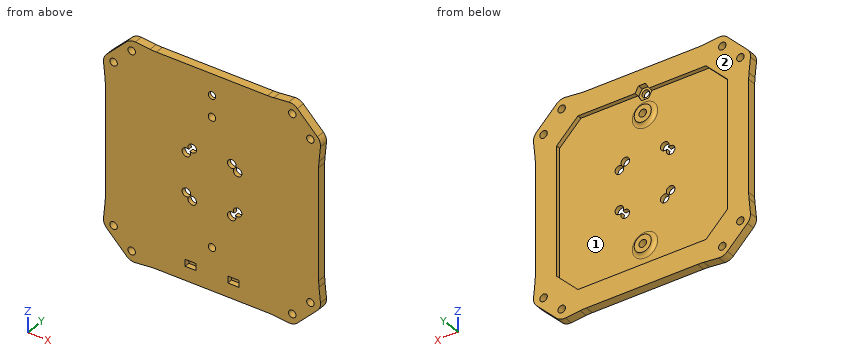
from build123d import *

# Parameters (mm, degrees)
SKETCH1_R                  = 1.75
BOSS_EXTRUDE1_DEPTH        = 4
CUT_EXTRUDE1_DEPTH         = 2
SKETCH4_R                  = 1.75
CUT_EXTRUDE3_DEPTH         = 73.238369544
BOSS_EXTRUDE2_START        = 1.5
SKETCH5_R                  = 4
SKETCH5_R_2                = 1.75
BOSS_EXTRUDE2_DEPTH        = 1.5
REDONDEO1_R                = 2
REDONDEO2_R                = 30
REDONDEO3_R                = 5
CORTAR_EXTRUIR2_DEPTH      = 2.5
CROQUIS1_R                 = 1.75
CORTAR_EXTRUIR1_DEPTH      = 5
CORTAR_EXTRUIR3_DEPTH      = 73.029377138
CORTAR_EXTRUIR3_DEPTH_BACK = 73.029377138
CROQUIS5_R                 = 2
CROQUIS6_W                 = 5.2
CROQUIS6_H                 = 3.2
CORTAR_EXTRUIR4_DEPTH      = 2.5


with BuildPart() as part:
    # Sketch1 → Boss-Extrude1 (new body)
    with BuildSketch(Plane(origin=(0, 0, 0), x_dir=(1, 0, 0), z_dir=(0, 1, 0))):
        Polygon((-27.516424079, 50), (27.516424079, 50), (38.33273811, 51.060660172), (51.060660172, 38.33273811), (50, 27.516424079), (50, -27.516424079), (51.060660172, -38.33273811), (38.33273811, -51.060660172), (27.516424079, -50), (-27.516424079, -50), (-38.33273811, -51.060660172), (-51.060660172, -38.33273811), (-50, -27.516424079), (-50, 27.516424079), (-51.060660172, 38.33273811), (-38.33273811, 51.060660172), align=None)
        with Locations(Location((37.625631329, 46.110912703, 0), (0, 0, 270))):
            Circle(SKETCH1_R, mode=Mode.SUBTRACT)
        with Locations(Location((46.110912703, 37.625631329, 0), (0, 0, 270))):
            Circle(SKETCH1_R, mode=Mode.SUBTRACT)
        with Locations(Location((37.625631329, -46.110912703, 0), (0, 0, 270))):
            Circle(SKETCH1_R, mode=Mode.SUBTRACT)
        with Locations(Location((46.110912703, -37.625631329, 0), (0, 0, 270))):
            Circle(SKETCH1_R, mode=Mode.SUBTRACT)
        with Locations(Location((-46.110912703, -37.625631329, 0), (0, 0, 270))):
            Circle(SKETCH1_R, mode=Mode.SUBTRACT)
        with Locations(Location((-37.625631329, -46.110912703, 0), (0, 0, 270))):
            Circle(SKETCH1_R, mode=Mode.SUBTRACT)
        with Locations(Location((-37.625631329, 46.110912703, 0), (0, 0, 270))):
            Circle(SKETCH1_R, mode=Mode.SUBTRACT)
        with Locations(Location((-46.110912703, 37.625631329, 0), (0, 0, 270))):
            Circle(SKETCH1_R, mode=Mode.SUBTRACT)
    extrude(amount=BOSS_EXTRUDE1_DEPTH)

    # Sketch2 → Cut-Extrude1 (cut)
    with BuildSketch(Plane(origin=(0, 4, 0), x_dir=(1, 0, 0), z_dir=(0, 1, 0))):
        Polygon((-40, -30), (-40, 30), (-30, 40), (30, 40), (40, 30), (40, -30), (30, -40), (-30, -40), align=None)
    extrude(amount=-CUT_EXTRUDE1_DEPTH, mode=Mode.SUBTRACT)

    # Sketch4 → Cut-Extrude3 (cut, through all)
    with BuildSketch(Plane(origin=(0, 2, 0), x_dir=(1, 0, 0), z_dir=(0, 1, 0))):
        with Locations(Location((0, 30, 0), (0, 0, 270))):
            Circle(SKETCH4_R)
    cut_extrude3 = extrude(amount=-CUT_EXTRUDE3_DEPTH, mode=Mode.SUBTRACT)

    # Sketch5 → Boss-Extrude2 (add)
    with BuildSketch(Plane(origin=(0, 2, 0), x_dir=(1, 0, 0), z_dir=(0, 1, 0)).offset(BOSS_EXTRUDE2_START)):
        with Locations(Location((0, 30, 0), (0, 0, 90))):
            Circle(SKETCH5_R)
        with Locations(Location((0, 30, 0), (0, 0, 270))):
            Circle(SKETCH5_R_2, mode=Mode.SUBTRACT)
    boss_extrude2 = extrude(amount=-BOSS_EXTRUDE2_DEPTH)

    # Simetría1: Cut-Extrude3, Boss-Extrude2 across plane
    add(cut_extrude3.mirror(Plane.XY), mode=Mode.SUBTRACT)
    add(boss_extrude2.mirror(Plane.XY))

    # Redondeo1
    # the kernel refuses this fillet: 2 mm, written as the material it adds along each edge
    with BuildSketch(Plane(origin=(0, 2, -30), x_dir=(0, 0, -1), z_dir=(1, 0, 0))) as redondeo1_piece_1:
        with BuildLine():
            CenterArc((5.936491673, 2), REDONDEO1_R, 194.477512186, 75.522487814)
            Line((4, 1.5), (3.961270167, 1.49))
            ThreePointArc((3.961270167, 1.49), (3.96, 0.75), (3.96, 0))
            Line((3.96, 0), (4, -0.04))
            Line((4, -0.04), (5.936491673, -0.04))
            Line((5.936491673, -0.04), (5.936491673, 0))
        make_face()
    revolve(axis=Axis((0, 2, -30), (0, 1, 0)))
    with BuildSketch(Plane(origin=(0, 2, 30), x_dir=(0, 0, 1), z_dir=(1, 0, 0))) as redondeo1_piece_2:
        with BuildLine():
            CenterArc((5.936491673, -2), REDONDEO1_R, 90, 75.522487814)
            Line((4, -1.5), (3.961270167, -1.49))
            ThreePointArc((3.961270167, -1.49), (3.96, -0.75), (3.96, 0))
            Line((3.96, 0), (4, 0.04))
            Line((4, 0.04), (5.936491673, 0.04))
            Line((5.936491673, 0.04), (5.936491673, 0))
        make_face()
    revolve(axis=Axis((0, 2, 30), (0, -1, 0)))

    # Redondeo2
    # the kernel refuses this fillet: 30 mm, written as the material it adds along each edge
    with BuildSketch(Plane(origin=(-27.516424079, 0, -50), x_dir=(1, 0, 0), z_dir=(0, 1, 0)), Plane(origin=(-27.516424079, 0, 50), x_dir=(-0.9952264052892461, 0, 0.09759304388656657), z_dir=(0, 1, 0)), Plane(origin=(-50, 0, 27.516424079), x_dir=(0, 0, -1), z_dir=(0, 1, 0)), Plane(origin=(-50, 0, -27.516424079), x_dir=(-0.09759304388655696, 0, -0.9952264052892469), z_dir=(0, 1, 0))) as redondeo2_piece_1:
        with BuildLine():
            CenterArc((REDONDEO2_R * 0.048913268002, REDONDEO2_R), REDONDEO2_R, 264.399415997, 5.600584003)
            Line((-REDONDEO2_R * 0.0486797758846, REDONDEO2_R * 0.00477359471075), (0, 0))
            Line((0, 0), (REDONDEO2_R * 0.048913268002, 0))
        make_face()
    extrude(amount=4)
    with BuildSketch(Plane(origin=(27.516424079, 0, -50), x_dir=(-1, 0, 0), z_dir=(0, 1, 0)), Plane(origin=(50, 0, -27.516424079), x_dir=(0.09759304388656798, 0, -0.9952264052892459), z_dir=(0, 1, 0)), Plane(origin=(50, 0, 27.516424079), x_dir=(0, 0, -1), z_dir=(0, 1, 0)), Plane(origin=(27.516424079, 0, 50), x_dir=(0.9952264052892461, 0, 0.09759304388656634), z_dir=(0, 1, 0))) as redondeo2_piece_2:
        with BuildLine():
            CenterArc((REDONDEO2_R * 0.048913268002, -REDONDEO2_R), REDONDEO2_R, 90, 5.600584003)
            Line((-REDONDEO2_R * 0.0486797758846, -REDONDEO2_R * 0.00477359471075), (0, 0))
            Line((0, 0), (REDONDEO2_R * 0.048913268002, 0))
        make_face()
    extrude(amount=4)

    # Redondeo3
    redondeo3_edges = [part.edges().sort_by_distance(p)[0] for p in [
        (38.33273811, 2, -51.060660172),
        (51.060660172, 2, -38.33273811),
        (51.060660172, 2, 38.33273811),
        (38.33273811, 2, 51.060660172),
        (-38.33273811, 2, 51.060660172),
        (-51.060660172, 2, 38.33273811),
        (-51.060660172, 2, -38.33273811),
        (-38.33273811, 2, -51.060660172),
    ]]
    fillet(redondeo3_edges, radius=REDONDEO3_R)

    # Croquis3 → Cortar-Extruir2 (cut)
    with BuildSketch(Plane(origin=(0, 4, 0), x_dir=(1, 0, 0), z_dir=(0, 1, 0))):
        Polygon((1.645448267, -37.15), (3.290896534, -40), (1.645448267, -42.85), (-1.645448267, -42.85), (-3.290896534, -40), (-1.645448267, -37.15), align=None)
    extrude(amount=-CORTAR_EXTRUIR2_DEPTH, mode=Mode.SUBTRACT)

    # Croquis1 → Cortar-Extruir1 (cut)
    with BuildSketch(Plane.XZ):
        with Locations(Location((0, 40, 0), (0, 0, 270))):
            Circle(CROQUIS1_R)
    extrude(amount=-CORTAR_EXTRUIR1_DEPTH, mode=Mode.SUBTRACT)

    # Croquis5 → Cortar-Extruir3 (cut, two sides: drawn at the far end of the back side and taken through both)
    with BuildSketch(Plane.XZ.offset(-CORTAR_EXTRUIR3_DEPTH_BACK)):
        with Locations((-12, -9.25)):
            Circle(CROQUIS5_R)
        with Locations((-12, 9.25)):
            Circle(CROQUIS5_R)
        with Locations((12, 9.25)):
            Circle(CROQUIS5_R)
        with Locations((12, -9.25)):
            Circle(CROQUIS5_R)
        with Locations((9.25, -12)):
            Circle(CROQUIS5_R)
        with Locations((-9.25, -12)):
            Circle(CROQUIS5_R)
        with Locations((9.25, 12)):
            Circle(CROQUIS5_R)
        with Locations((-9.25, 12)):
            Circle(CROQUIS5_R)
    extrude(amount=CORTAR_EXTRUIR3_DEPTH + CORTAR_EXTRUIR3_DEPTH_BACK, mode=Mode.SUBTRACT)

    # Croquis6 → Cortar-Extruir4 (cut)
    with BuildSketch(Plane.XZ):
        with Locations((-10, -41.9)):
            Rectangle(CROQUIS6_W, CROQUIS6_H)
        with Locations((10, -41.9)):
            Rectangle(CROQUIS6_W, CROQUIS6_H)
    extrude(amount=-CORTAR_EXTRUIR4_DEPTH, mode=Mode.SUBTRACT)


solid = part.part
Read the model definition and answer for the solid it produces. Units are mm, in the model's axes. Face numbers are marked on the shaded views. Round coordinates to 2 decimals unless told otherwise and drop trailing zeros. Order: outer loops, then holes, each group sorted by start corner. A loop starts at its lowest first (then second) coordinate and runs counter-clockwise, first axis right, second up.
1) The part is cut by section A-A on x = 0. Give the number of separate pieces and of enclosed holes in the cut face, plus the area to 3 significant figures.
2) The part is cut by section B-B on x = -34.5. Write down the section's boundary in (y, z), plus the area to 3 significant figures.
3) Flat-ended cylindrical pins translate along their axes: pin 1 (1 mm diameter, centred on x = -18, y = 2.5, fed in from -Z); pin 2 (1.5 mm diameter, centred on y = 2.5, z = 23, fed in from -X); pin 3 (6.5 mm diameter, centred on x = 12, z = 9.25, fed in from +Y); pin 4 (3 mm diameter, centred on x = 0, z = 40, fed in from -Y). Find the tip coordinate at first contact, or state that the pin passes through.
4) The mould has two halves that part along X. Classify the marked faces 1 and 2: released by +X, released by -X, zero draft, split by the parting line, or undercut.
5) Straight lines are drawn through the part: L1, parallel to X at y = 1.5, z = -12; L2, parallel to Z at x = -9.5, y = 1.1; L3, parallel to X at y = 1.3, z = 9.25. For each, find the intervals that lie inside material, in ascending order.
Resolved:
1. separate pieces: 4
1. enclosed holes: 0
1. area: 229 mm2
2. outline: (0, -50.68) - (4, -50.68) - (4, -35.5) - (2, -35.5) - (2, 35.5) - (4, 35.5) - (4, 50.68) - (0, 50.68) - close
2. area: 263 mm2
3. pin 1: stops at z = -50
3. pin 2: stops at x = -50
3. pin 3: stops at y = 2
3. pin 4: passes through
4. face 1: undercut
4. face 2: zero draft
5. L1: x = -50 to -11.25, -7.25 to 7.25, 11.25 to 50
5. L2: z = -50 to -43.5, -40.3 to -13.98, -10.02 to 10.02, 13.98 to 50
5. L3: x = -50 to -14, -10 to 10, 14 to 50
